The model under review builds one solid part; all positions refer to its coordinate system, in mm. Face numbers are marked on the shaded views. A direction names the side the tool comes from. Round coordinates to 2 decimals unless told otherwise and drop trailing zeros. Order: outer loops, then holes, each group sorted by start corner. A loop starts at its lowest first (then second) coordinate and runs counter-clockwise, first axis right, second up. Notation, with made-up numbers: M 72.5,87 L 105.5,87 A30 cw 105.5,120 Z; hole C 55.5,12.25 d6. An arc over 180 degrees is marked long. Use a Markdown table: item, result. Add a question column.
1. For the marked faces 1, 2, 3, 4 and 5, list the 3-axis set-ups (+Z, -Z, +X, -X, +Y, -Y) from which the entire face can be reached by the end or side of a thin tool; tool diameter is ignored.
2. Consider section B-B on z = 0. State the section outline as (x, y) points (3 decimals).
3. Consider section D-D on z = 9. State the section outline as (x, y) points, then the cut area to 3 significant figures.
4. Consider section A-A on x = 0. State the section outline as (y, z) points (3 decimals), then the cut area to 3 significant figures.
5. Insertion check: P1, Ø4.5, axis at y = -3, z = -3.5, coming from the -X side (3 decimals); P2, Ø8, axis at x = 11.5, y = -48, coming from the +Z side; P3, Ø1.5, axis at x = 17, z = -3.5, coming from the -Y side. Each pin has a flat end and moves straight along its axis. Give the tip position at first contact, or say it passes through.
6. Consider section C-C on y = -7. State the section outline as (x, z) points (3 decimals), then the cut area to 3 significant figures.
7. To check wall thickness, follow probe 1 along Y at (x, z) = (6, -15); probe 2 along Z at (x, y) = (8, -43); probe 3 along X at (y, z) = (-50, 5.5). State the ranges of each line that lie inside material, in increasing order.
8. The part is to be moulded in two halves that separate along Z. For the marked faces 6, 7 and 8, say which applies: +Z half, -Z half, draft (parallel to the pull), parting line (faces both ways), or undercut.
from build123d import *

# Parameters (mm, degrees)
CYLINDER_R          = 17.78
CYLINDER_DEPTH      = 76.2
CYLINDER_ROLL_ANGLE = 90
SKETCH_R            = 13.335
POCKET_DEPTH        = 76.2
SKETCH001_R         = 19.05
POCKET001_DEPTH     = 8.89
SKETCH002_R         = 19.05
POCKET002_DEPTH     = 8.89


with BuildPart() as part:
    # Cylinder → Cylinder (new body)
    with BuildSketch(Plane.XY):
        Circle(CYLINDER_R)
    extrude(amount=CYLINDER_DEPTH)


with BuildPart() as part_1:
    # Cylinder roll: moved
    add(part.part.rotate(Axis((0, 0, 0), (1, 0, 0)), CYLINDER_ROLL_ANGLE))


with BuildPart() as part_2:
    # Cylinder placement: moved
    add(part_1.part)

    # Sketch → Pocket (cut)
    with BuildSketch(Plane(origin=(0, 0, 0), x_dir=(1, 0, 0), z_dir=(0, 1, 0))):
        Circle(SKETCH_R)
    extrude(amount=-POCKET_DEPTH, mode=Mode.SUBTRACT)

    # Sketch001 → Pocket001 (cut)
    with BuildSketch(Plane(origin=(0, 0, 0), x_dir=(1, 0, 0), z_dir=(0, 1, 0))):
        Circle(SKETCH001_R)
        Polygon((-15.875, -9.165436), (-15.875, 9.165436), (0, 18.330871), (15.875, 9.165436), (15.875, -9.165436), (0, -18.330871), align=None, mode=Mode.SUBTRACT)
    extrude(amount=-POCKET001_DEPTH, mode=Mode.SUBTRACT)

    # Sketch002 → Pocket002 (cut)
    with BuildSketch(Plane.XZ.offset(76.2)):
        Circle(SKETCH002_R)
        Polygon((-15.875, -9.165436), (-15.875, 9.165436), (0, 18.330871), (15.875, 9.165436), (15.875, -9.165436), (0, -18.330871), align=None, mode=Mode.SUBTRACT)
    extrude(amount=-POCKET002_DEPTH, mode=Mode.SUBTRACT)


solid = part_2.part
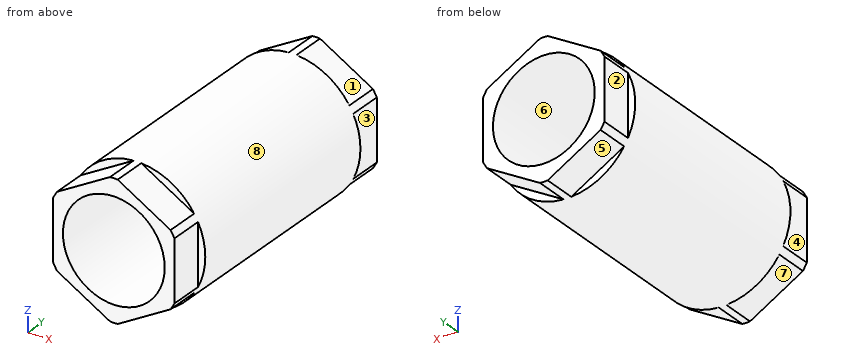
Answer block:
| question | item | result |
|---|---|---|
| 1 | face 1 | +Z, +X, +Y |
| 1 | face 2 | +Z, -Z, -X, +Y |
| 1 | face 3 | +Z, -Z, +X, +Y |
| 1 | face 4 | +Z, -Z, -X, -Y |
| 1 | face 5 | -Z, -X, +Y |
| 2 | outline | M -17.78,-67.31 L -15.875,-67.31 L -15.875,-76.2 L -13.335,-76.2 L -13.335,0 L -15.875,0 L -15.875,-8.89 L -17.78,-8.89 Z; M 13.335,-76.2 L 15.875,-76.2 L 15.875,-67.31 L 17.78,-67.31 L 17.78,-8.89 L 15.875,-8.89 L 15.875,0 L 13.335,0 Z |
| 3 | outline | M -15.33,-76.2 L -9.84,-76.2 L -9.84,0 L -15.33,0 Z; M 9.84,-76.2 L 15.33,-76.2 L 15.33,0 L 9.84,0 Z |
| 3 | area | 837 mm^2 |
| 4 | outline | M -76.2,-17.78 L 0,-17.78 L 0,-13.335 L -76.2,-13.335 Z; M -76.2,13.335 L 0,13.335 L 0,17.78 L -76.2,17.78 Z |
| 4 | area | 677 mm^2 |
| 5 | P1 | x = -15.875 |
| 5 | P2 | z = 16.12 |
| 5 | P3 | y = -67.31 |
| 6 | outline | M -15.875,-8.007 A17.78 ccw -14.872,-9.745 L -1.003,-17.752 A17.78 ccw 1.003,-17.752 L 14.872,-9.745 A17.78 ccw 15.875,-8.007 L 15.875,8.007 A17.78 ccw 14.872,9.745 L 1.003,17.752 A17.78 ccw -1.003,17.752 L -14.872,9.745 A17.78 ccw -15.875,8.007 Z; hole C 0,0 d26.67 |
| 6 | area | 311 mm^2 |
| 7 | probe 1 | -67.31 to -8.89 |
| 7 | probe 2 | -15.88 to -10.67, 10.67 to 15.88 |
| 7 | probe 3 | -16.91 to -12.15, 12.15 to 16.91 |
| 8 | face 6 | undercut |
| 8 | face 7 | -Z half |
| 8 | face 8 | parting line |
